from build123d import *

# Parameters (mm, degrees)
F1_DEPTH = 24
F2_R     = 1.7
F3_DEPTH = 25


# Not quite as in the source:
# - a feature names something its author has since deleted; it is built from what else it names


with BuildPart() as f1:
    # F0 (on Front) → F1 (new body)
    with BuildSketch(Plane.XZ):
        with BuildLine():
            ThreePointArc((-7.7, 0), (0, 7.7), (7.7, 0))
            Line((7.7, 0), (15.7, 0))
            Line((15.7, 0), (27.7, 0))
            Line((27.7, 0), (27.7, 6))
            Line((27.7, 6), (14.5082735017, 6))
            ThreePointArc((14.5082735017, 6), (0, 15.7), (-14.5082735017, 6))
            Line((-14.5082735017, 6), (-27.7, 6))
            Line((-27.7, 6), (-27.7, 0))
            Line((-27.7, 0), (-15.7, 0))
            Line((-15.7, 0), (-7.7, 0))
        make_face()
    extrude(amount=F1_DEPTH)

    # F2 (on face) → F3 (cut)
    with BuildSketch(Plane.XY.offset(6)):
        with Locations((-21.7, -12)):
            Circle(F2_R)
        with Locations((21.7, -12)):
            Circle(F2_R)
    extrude(amount=-F3_DEPTH, mode=Mode.SUBTRACT)


solid = f1.part
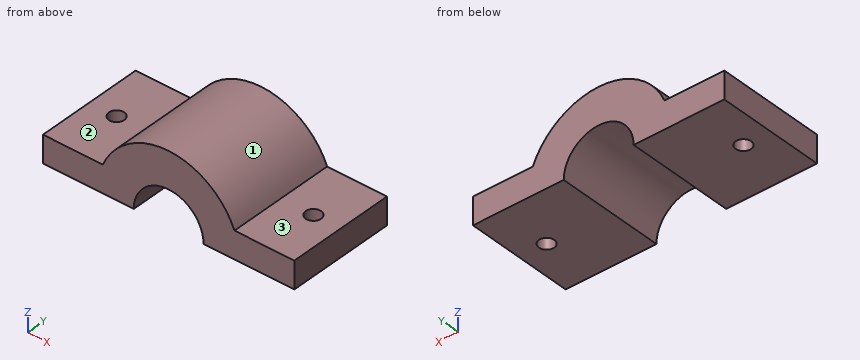
Read the model definition and answer for the solid it produces. Units are mm, in the model's axes. Face numbers are marked on the shaded views. A direction names the side the tool comes from. Coordinates: 2 decimals unless noted, no trailing zeros. Write each loop counter-clockwise with the first axis right and the second up, starting at its lowest first coordinate (ties: lowest second). Pieces come first, ordered by that corner, then holes. Notation, with made-up numbers: M 24,11 L 72,11 A25 cw 72,36 Z; hole C 29.25,66 d1. An arc over 180 degrees is marked long. Use a Markdown table: item, result.
Q1. The part is cut by section D-D, the plane y = -20.25. Write down the section's boundary in (x, z).
Answer block:
| item | result |
|---|---|
| outline | M -27.7,0 L -7.7,0 A7.7 cw 7.7,0 L 27.7,0 L 27.7,6 L 14.51,6 A15.7 ccw -14.51,6 L -27.7,6 Z |
Q2. Straight lines are drawn through the part: L1, parallel to Y at x = 21.7, z = 3.5; L2, parallel to Z at x = 17.5, y = -17.5; L3, parallel to X at y = -6, z = 6.75. For each, find the intervals that lie inside material, in ascending order. Write a range as [from, to].
Answer block:
| item | result |
|---|---|
| L1 | y = [-24, -13.7], [-10.3, 0] |
| L2 | z = [0, 6] |
| L3 | x = [-14.17, -3.71], [3.71, 14.17] |
Q3. The part is cut by section B-B, the plane z = 1.5. Write down the section's boundary in (x, y), then the cut area to 3 significant figures.
Answer block:
| item | result |
|---|---|
| outline | M -27.7,-24 L -7.55,-24 L -7.55,0 L -27.7,0 Z; M 7.55,-24 L 27.7,-24 L 27.7,0 L 7.55,0 Z; hole C -21.7,-12 d3.4; hole C 21.7,-12 d3.4 |
| area | 949 mm2 |
Q4. The part is cut by section C-C, the plane x = -21.7. Write down the section's boundary in (y, z).
Answer block:
| item | result |
|---|---|
| outline | M -24,0 L -13.7,0 L -13.7,6 L -24,6 Z; M -10.3,0 L 0,0 L 0,6 L -10.3,6 Z |
Q5. The part is cut by section A-A, the plane y = -12. Write down the section's boundary in (x, z), then the cut area to 3 significant figures.
Answer block:
| item | result |
|---|---|
| outline | M -27.7,0 L -23.4,0 L -23.4,6 L -27.7,6 Z; M -20,0 L -7.7,0 A7.7 cw 7.7,0 L 20,0 L 20,6 L 14.51,6 A15.7 ccw -14.51,6 L -20,6 Z; M 23.4,0 L 27.7,0 L 27.7,6 L 23.4,6 Z |
| area | 402 mm2 |
Q6. Which of the six approach directions +Z, -Z, +X, -X, +Y, -Y give full straight-line access (tool end or side, diameter ignored) to the marked faces 1, 2 and 3?
Answer block:
| item | result |
|---|---|
| face 1 | +Z, +Y, -Y |
| face 2 | +Z, -X, +Y, -Y |
| face 3 | +Z, +X, +Y, -Y |
Q7. Each of these flat-tipped pins is pushed along its axis until it touches: pin 1 Ø6 at (x, y) = (-10.5, -7) entering from +Z; pin 2 Ø1 at (y, z) = (-4, 10) entering from -X; pin 3 Ø1 at (y, z) = (-8, 9.5) entering from +X. Where does it stop, or does it pass through?
Answer block:
| item | result |
|---|---|
| pin 1 | stops at z = 13.79 |
| pin 2 | stops at x = -12.5 |
| pin 3 | stops at x = 12.86 |
